Work out the finished part from the listing and answer in its coordinate system (mm). Face numbers are marked on the shaded views. A direction names the side the tool comes from. Give positions to 0.01 mm unless a question says otherwise; leave off trailing zeros. Loops run counter-clockwise (first coordinate to the right, second up) from the corner with the lowest first, then second, coordinate; pieces in that order, holes last. Notation, with made-up numbers: M 78.5,62.5 L 127.5,62.5 A23 ccw 127.5,79.5 Z; hole C 83.25,-3 d4. An arc over 180 degrees is marked long. Answer as a JSON object with one key per item and string values. Group by question number.
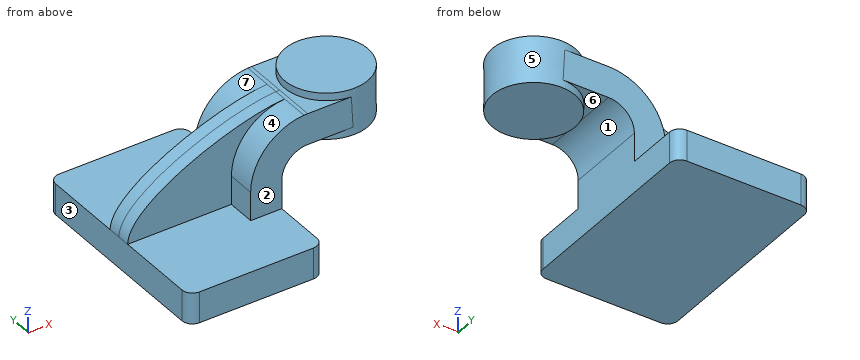
```python
from build123d import *

# Parameters (mm, degrees)
F1_DEPTH = 63.5
F2_DEPTH = 7.9375
F3_DEPTH = 25.4
F0_W     = 25.3238
F0_H     = 19.05
F4_DEPTH = 25.4
F6_R     = 6.35


with BuildPart() as f1:
    # F0 (on Front) → F1 (new body, symmetric)
    with BuildSketch(Plane.XZ):
        Polygon((-41.275, 9.525), (-41.275, -9.525), (41.275, -9.525), (41.275, 9.525), (22.225, 9.525), align=None)
    extrude(amount=F1_DEPTH, both=True)

    # F0 (on Front) → F2 (join, symmetric)
    with BuildSketch(Plane.XZ):
        with BuildLine():
            add(Edge.make_bspline(
                [(-41.275, 9.525), (-41.0096709394, 33.3485221213), (24.4764054446, 60.2335256768), (54.8747860488, 61.8510109874)],
                knots=[0, 0, 0, 0, 108.7072951775, 108.7072951775, 108.7072951775, 108.7072951775], degree=3))
            Line((-41.275, 9.525), (22.225, 9.525))
            Line((22.225, 9.525), (22.225, 27.0002))
            ThreePointArc((22.225, 27.0002), (31.6625769031, 50.8779488235), (54.8747860488, 61.8510109874))
        make_face()
    extrude(amount=F2_DEPTH, both=True)

    # F0 (on Front) → F3 (join, symmetric)
    with BuildSketch(Plane.XZ):
        with BuildLine():
            Line((22.225, 9.525), (41.275, 9.525))
            Line((41.275, 9.525), (41.275, 27.0002))
            ThreePointArc((41.275, 27.0002), (45.9246798487, 38.2255201513), (57.15, 42.8752))
            Line((57.15, 42.8752), (60.325, 42.8752))
            Line((60.325, 42.8752), (60.325, 61.9252))
            Line((60.325, 61.9252), (57.15, 61.9252))
            add(Edge.make_bspline(
                [(54.8747860488, 61.8510109874), (55.6569929467, 61.8926318942), (56.4159672755, 61.917522453), (57.15, 61.9252)],
                knots=[108.7072951775, 108.7072951775, 108.7072951775, 108.7072951775, 111.5045361635, 111.5045361635, 111.5045361635, 111.5045361635], degree=3))
            ThreePointArc((54.8747860488, 61.8510109874), (31.6625769031, 50.8779488235), (22.225, 27.0002))
            Line((22.225, 27.0002), (22.225, 9.525))
        make_face()
    extrude(amount=F3_DEPTH, both=True)

    # F0 (on Front) → F4 (join, symmetric)
    with BuildSketch(Plane.XZ):
        with Locations((72.9869, 52.4002)):
            Rectangle(F0_W, F0_H)
    extrude(amount=F4_DEPTH, both=True)

    # F0 (on Front) → F5 (revolve)
    with BuildSketch(Plane.XZ):
        Polygon((111.125, 66.675), (85.6488, 66.675), (85.725, 38.1), (111.125, 38.1), align=None)
    revolve(axis=Axis((85.6869, 0, 52.3875), (-0.0026666572, 0, 0.9999964445)))

    # F6
    f6_edges = [f1.edges().sort_by_distance(p)[0] for p in [
        (41.275, -63.5, 0),
        (41.275, 63.5, 0),
        (-41.275, 63.5, 0),
        (-41.275, -63.5, 0),
    ]]
    fillet(f6_edges, radius=F6_R)


solid = f1.part
```
Item 1: For a pull along X with two mould halves and no side action, classify the marked faces 1, 2 and 3 as pulls with the +X half, pulls with the -X half, needs draft (parallel to the pull), parting line crosses it, or undercut.
Item 2: Find the intervals of material crossed by probe 1 along Y at (x, z) = (16, 51.5); probe 2 along Z at (x, y) = (-32, 12) (3 decimals); probe 3 along Y at (x, z) = (29, 41), in increasing order. Write a range as [from, to].
Item 3: A tool of negligible diameter and unlimited length cuts with its end or side. For the marked faces 4, 5, 6 and 7, from which of +Z, -Z, +X, -X, +Y, -Y can it reach the whole face along a straight path? Write none if from no direction.
Item 4: A cutting plane is placed at A-A (z = -4). Determine the outline of the cut face in (x, y) (3 decimals).
Item 5: A cutting plane is placed at B-B (y = 32). Determine the outline of the cut face in (x, z) (3 decimals), and give its area (3 significant figures).
Item 6: Given pin 1 Ø8 at (x, z) = (5, 45) entering from -Y; pin 2 Ø15.5 at (x, z) = (42.5, 23) entering from +Y; pin 3 Ø8 at (x, z) = (65, 38) entering from +Y, each flat-ended and moving along its own axis, determine where each tip first touches the part or whether it passes through.
The answers:
{
 "1": {"face 1": "undercut", "face 2": "needs draft", "face 3": "pulls with the -X half"},
 "2": {"probe 1": "y = [-7.94, 7.94]", "probe 2": "z = [-9.525, 9.525]", "probe 3": "y = [-25.4, 25.4]"},
 "3": {"face 4": "+Z, -X, -Y", "face 5": "none", "face 6": "-Z", "face 7": "+Z, -X, +Y"},
 "4": {"outline": "M -41.275,-57.15 A6.35 ccw -34.925,-63.5 L 34.925,-63.5 A6.35 ccw 41.275,-57.15 L 41.275,57.15 A6.35 ccw 34.925,63.5 L -34.925,63.5 A6.35 ccw -41.275,57.15 Z"},
 "5": {"outline": "M -41.275,-9.525 L 41.275,-9.525 L 41.275,9.525 L -41.275,9.525 Z", "area": "1,570 mm^2"},
 "6": {"pin 1": "stops at y = -7.94", "pin 2": "stops at y = 25.4", "pin 3": "stops at y = 19.12"}
}
